The listing builds one solid part. Answer for the finished solid, in the listing's coordinates (mm). A direction names the side the tool comes from. Coordinates: 2 decimals unless noted, no trailing zeros. Order: outer loops, then holes, each group sorted by start corner. A loop starts at its lowest first (then second) coordinate and runs counter-clockwise, first axis right, second up.
from build123d import *

# Parameters (mm, degrees)
SKETCH1_R           = 4.7625
BOSS_EXTRUDE1_DEPTH = 6.35


with BuildPart() as part:
    # Sketch1 → Boss-Extrude1 (new body)
    with BuildSketch(Plane.XY):
        with BuildLine():
            Line((-82.55, -12.7), (0, -12.7))
            ThreePointArc((0, -12.7), (12.7, 0), (0, 12.7))
            Line((0, 12.7), (-69.85, 12.7))
            Line((-69.85, 12.7), (-69.85, 50.8))
            ThreePointArc((-69.85, 50.8), (-82.55, 63.5), (-95.25, 50.8))
            Line((-95.25, 50.8), (-95.25, 0))
            ThreePointArc((-95.25, 0), (-91.530256121, -8.980256121), (-82.55, -12.7))
        make_face()
        with Locations((-82.55, 12.7)):
            Circle(SKETCH1_R, mode=Mode.SUBTRACT)
        Circle(SKETCH1_R, mode=Mode.SUBTRACT)
        with Locations((-82.55, 0)):
            Circle(SKETCH1_R, mode=Mode.SUBTRACT)
        with Locations((-82.55, 50.8)):
            Circle(SKETCH1_R, mode=Mode.SUBTRACT)
        with Locations((-82.55, 25.4)):
            Circle(SKETCH1_R, mode=Mode.SUBTRACT)
    extrude(amount=BOSS_EXTRUDE1_DEPTH)


solid = part.part
1) Section D-D (y = 10.5) is taken. Give the vertices of the cut face in (x, z).
2) Section C-C (x = -86) is taken. Give the vertices of the cut face in (y, z).
3) Consider L1, parallel to Y at x = -82.55, z = 4; L2, parallel to Y at x = -47, z = 4.25; L3, parallel to X at y = 31, z = 4.75. Determine where each line is inside the solid, lowest interval first.
4) A tool of negligible diameter and unlimited length cuts with its end or side. For faces 1 (the face through (-69.85, 31, 3)), 2 (the face through (-95.25, 26, 3)), from which of +Z, -Z, +X, -X, +Y, -Y can it reach the whole face along a straight path? Write none if from no direction.
5) Section B-B (z = 1.25) is taken. Give the number of separate pieces and of enclosed holes in the cut face, then the cut area to 3 significant figures.
6) Each of these flat-tipped pins is pushed along its axis until it touches: P1, Ø12.5, axis at x = -82.55, y = 12.7, coming from the -Z side; P2, Ø2, axis at x = -79, z = 2, coming from the +Y side; P3, Ø1, axis at x = -46, z = 3, coming from the +Y side; P4, Ø1.9, axis at y = 23, z = 3.5, coming from the +X side. Where does it stop, or does it pass through?
7) Section A-A (y = 25.4) is taken. Give the vertices of the cut face in (x, z).
8) Determine the mould class of faces 3 (the face through (-34, 12.7, 3)), 4 (the face through (-78.15, 10.88, 3.13)), 5 (the face through (-82.271, 63.497, 3.131)) for opening direction X: released by +X, released by -X, zero draft, split by the parting line, or undercut.
Filled sheet:
1. outline: (-95.25, 0) - (-86.77, 0) - (-86.77, 6.35) - (-95.25, 6.35) - close; (-78.33, 0) - (7.14, 0) - (7.14, 6.35) - (-78.33, 6.35) - close
2. outline: (-12.22, 0) - (-3.28, 0) - (-3.28, 6.35) - (-12.22, 6.35) - close; (3.28, 0) - (9.42, 0) - (9.42, 6.35) - (3.28, 6.35) - close; (15.98, 0) - (22.12, 0) - (22.12, 6.35) - (15.98, 6.35) - close; (28.68, 0) - (47.52, 0) - (47.52, 6.35) - (28.68, 6.35) - close; (54.08, 0) - (63.02, 0) - (63.02, 6.35) - (54.08, 6.35) - close
3. L1: y = -12.7 to -4.76, 4.76 to 7.94, 17.46 to 20.64, 30.16 to 46.04, 55.56 to 63.5
3. L2: y = -12.7 to 12.7
3. L3: x = -95.25 to -69.85
4. face 1: +Z, -Z, +X, +Y
4. face 2: +Z, -Z, -X, +Y, -Y
5. separate pieces: 1
5. enclosed holes: 5
5. area: 3,500 mm2
6. P1: stops at z = 0
6. P2: stops at y = 63.24
6. P3: stops at y = 12.7
6. P4: stops at x = -69.85
7. outline: (-95.25, 0) - (-87.31, 0) - (-87.31, 6.35) - (-95.25, 6.35) - close; (-77.79, 0) - (-69.85, 0) - (-69.85, 6.35) - (-77.79, 6.35) - close
8. face 3: zero draft
8. face 4: undercut
8. face 5: split by the parting line
